Autodesk Inventor part; units mm, degrees
ref_plane "YZ Plane" through (0, 0, 0) normal (1, 0, 0) x (0, 1, 0)
ref_plane "XZ Plane" through (0, 0, 0) normal (0, 1, 0) x (-1, 0, 0)
ref_plane "XY Plane" through (0, 0, 0) normal (0, 0, 1) x (1, 0, 0)
sketch "Sketch1" plane through (0, 0, 0) normal (0, 1, 0) x (-1, 0, 0)
  circle A0 centre (0, 0) radius 6
  circle A1 centre (0, 0) radius 8.5
  line L0 (12.5, 12) -> (-12.5, 12)
  line L1 (-12.5, 12) -> (-12.5, 6)
  line L2 (-12.5, 6) -> (12.5, 6)
  line L3 (12.5, 6) -> (12.5, 12)
  line L4 (12.5, 9) -> (-12.5, 9) construction
  circle A2 centre (8.5, 9) radius 1.625
  circle A3 centre (-8.5, 9) radius 1.625
  dimension "d0" = 12
  dimension "d1" = 17
  dimension "d2" = 25
  dimension "d3" = 6
  dimension "d4" = 12.5
  dimension "d5" = 3.25
  dimension "d6" = 3.25
  dimension "d7" = 17
  dimension "d8" = 4
extrude "Extrusion1" add sketch "Sketch1" along normal blind 5
chamfer "Chamfer2" distance 2.5 angle 45 2 edges at (-12.5, 2.5, 6) (12.5, 2.5, 6)
fillet "Fillet3" radius 1 24 edges at (8.0104, 0, 6) (11.25, 0, 7.25) (12.5, 0, 10.25) (0, 0, 12) (-12.5, 0, 10.25) (-8.0104, 0, 6) (-10, 2.5, 6) (-12.5, 5, 10.25) (-12.5, 2.5, 8.5) (-11.25, 5, 7.25) (-8.0104, 5, 6) (-11.25, 0, 7.25) (-6.0208, 2.5, 6) (6.0208, 2.5, 6) (0, 0, -8.5) (0, 5, -8.5) (8.0104, 5, 6) (10, 2.5, 6) (11.25, 5, 7.25) (12.5, 5, 10.25) (0, 5, 12) (-12.5, 2.5, 12) (12.5, 2.5, 8.5) (12.5, 2.5, 12)
equation "\"d8\" = -0.5 * d7 + 0.5 * d2"
properties part number "proxymity_holder_v2" material "ABS Plastic"
Part model, mm, in its own coordinate system. A direction names the side the tool comes from. Give positions to 0.01 mm unless a question says otherwise; leave off trailing zeros. Write each loop counter-clockwise with the first axis right and the second up, starting at its lowest first coordinate (ties: lowest second). Pieces come first, ordered by that corner, then holes. Notation, with made-up numbers: (-24.75, 27) -> (13.25, 27) arc R21 cw to (13.25, 52) -> close; hole circle Ø7 at (6.5, 61.5). An arc over 180 degrees is marked (long way). Put each result on its own line as item: value. Start each with the question number.
Item 1: Cut at D-D (y = 2.5). List the corners of the cut face in (x, z) (3 decimals), then the cut area to 4 significant figures.
Item 2: Wall check: L1, parallel to Z at x = -7.5, y = 4.6; L2, parallel to X at y = 3.3, z = 0; L3, parallel to X at y = 4, z = 10. Give the ranges that are in metal, low to high. Write a range as [from, to].
Item 3: Cut at C-C (z = 7.75). State how many separate pieces and enclosed holes the cut face has, then the cut area to 3 significant figures.
Item 4: Which spindle directions (+Z, -Z, +X, -X, +Y, -Y) get a long thin tool onto all of the face, cutting with end or side? Do faces 4 (the face through (0, 2, 12)), 5 (the face through (9, 2, 6)). Say none if no direction does.
Item 5: Cut at A-A (z = 0). List the corners of the cut face in (x, y), then the cut area to 3 significant figures.
Item 6: Pull direction Z, two halves, no side cores. Call faces 1 (the face through (11.051, 0.285, 7.476)), 2 (the face through (-12.215, 2.521, 11.699)), 3 (the face through (-8.29, 2.46, 7.39)): pulls with the +Z half, pulls with the -Z half, needs draft (parallel to the pull), parting line crosses it, or undercut.
Item 7: Pin check, flat tips, straight feed: pin 1 Ø1.5 at (x, z) = (9.5, 5) entering from -Y; pin 2 Ø1.5 at (x, y) = (-6.5, 1.5) entering from -Z; pin 3 Ø2 at (y, z) = (2, -1.5) entering from +X. Stop position of each tip, or through.
Item 8: Cut at B-B (y = 0.6). List the corners of the cut face in (x, z) (3 decimals), then the cut area to 3 significant figures.
Answer list:
1. outline: (-12.5, 8.914) arc R1 ccw to (-12.207, 8.207) -> (-10.293, 6.293) arc R1 ccw to (-9.586, 6) -> (-8.078, 6) arc R1 cw to (-7.227, 4.474) arc R8.5 ccw (long way) to (7.227, 4.474) arc R1 cw to (8.078, 6) -> (9.586, 6) arc R1 ccw to (10.293, 6.293) -> (12.207, 8.207) arc R1 ccw to (12.5, 8.914) -> (12.5, 11) arc R1 ccw to (11.5, 12) -> (-11.5, 12) arc R1 ccw to (-12.5, 11) -> close; hole circle Ø3.25 at (-8.5, 9); hole circle Ø12 at (0, 0); hole circle Ø3.25 at (8.5, 9)
1. area: 221.5 mm2
2. L1: z = [-3.56, 3.56], [6.05, 7.72], [10.28, 11.8]
2. L2: x = [-8.5, -6], [6, 8.5]
2. L3: x = [-12.5, -9.78], [-7.22, 7.22], [9.78, 12.5]
3. separate pieces: 3
3. enclosed holes: 0
3. area: 95.5 mm2
4. face 4: +Z, +X, -X, +Y, -Y
4. face 5: +X, +Y, -Y
5. outline: (-8.5, 1) arc R1 ccw to (-7.5, 0) -> (-6, 0) -> (-6, 5) -> (-7.5, 5) arc R1 ccw to (-8.5, 4) -> close; (6, 0) -> (7.5, 0) arc R1 ccw to (8.5, 1) -> (8.5, 4) arc R1 ccw to (7.5, 5) -> (6, 5) -> close
5. area: 24.1 mm2
6. face 1: pulls with the -Z half
6. face 2: pulls with the +Z half
6. face 3: undercut
7. pin 1: passes through
7. pin 2: stops at z = -6.26
7. pin 3: stops at x = 8.49
8. outline: (-12.417, 8.914) arc R0.917 ccw to (-12.148, 8.266) -> (-10.234, 6.352) arc R0.917 ccw to (-9.586, 6.083) -> (-8.078, 6.083) arc R1.083 cw to (-7.156, 4.43) arc R8.417 ccw (long way) to (7.156, 4.43) arc R1.083 cw to (8.078, 6.083) -> (9.586, 6.083) arc R0.917 ccw to (10.234, 6.352) -> (12.148, 8.266) arc R0.917 ccw to (12.417, 8.914) -> (12.417, 11) arc R0.917 ccw to (11.5, 11.917) -> (-11.5, 11.917) arc R0.917 ccw to (-12.417, 11) -> close; hole circle Ø3.25 at (-8.5, 9); hole circle Ø12 at (0, 0); hole circle Ø3.25 at (8.5, 9)
8. area: 215 mm2
